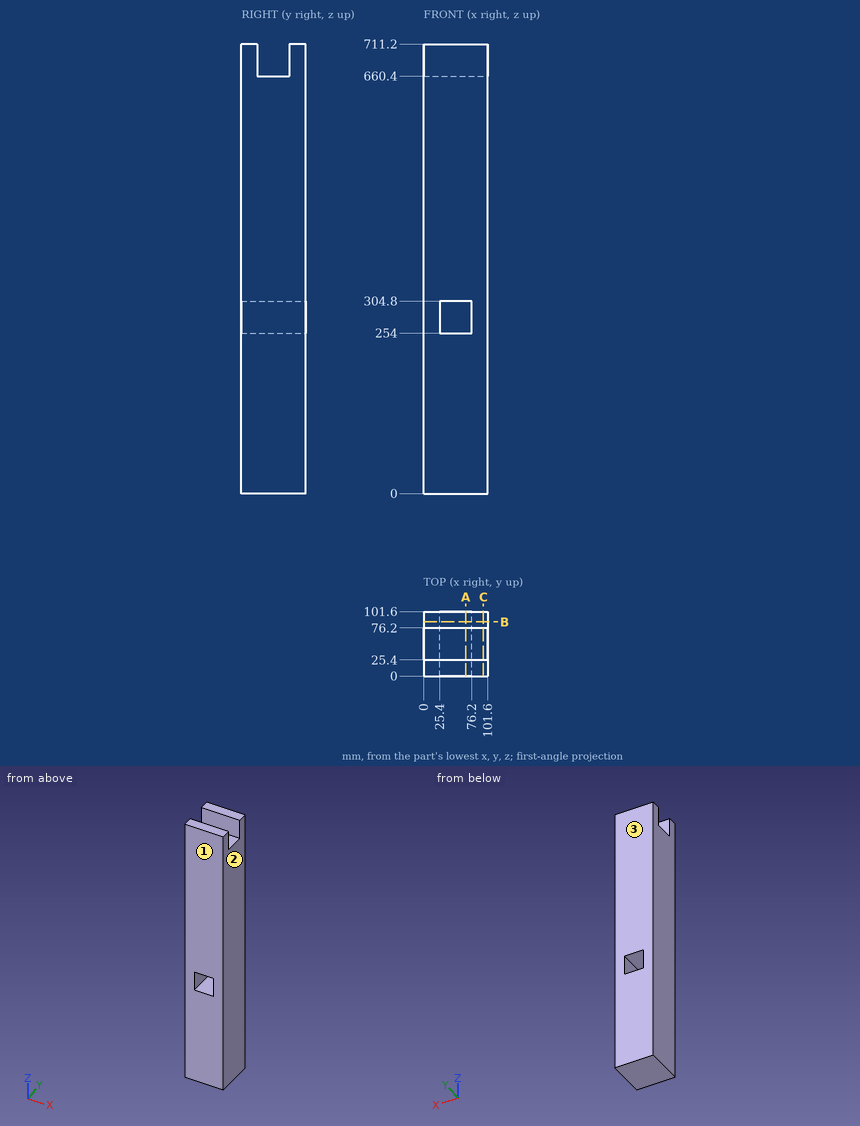
Part print with two shaded views. Sizes in mm from the minimum x, y, z corner. Round coordinates to 2 decimals unless told otherwise and drop trailing zeros. Loops run counter-clockwise (first coordinate to the right, second up) from the corner with the lowest first, then second, coordinate; pieces in that order, holes last. Notation, with made-up numbers: M 7.5,-4 L 27.5,-4 A12 cw 27.5,13 Z; hole C -30,15 d7. An arc over 180 degrees is marked long. Return JSON: item names as keys, results as strings. Group by question number.
(1) Saw through at B-B, the plane y = 85.5. List the corners of the cut face in (x, z), and give its area (3 significant figures).
(2) Mould opens along Y. For the marked faces 1, 2 and 3 say: +Y half, -Y half, draft (parallel to the pull), parting line (faces both ways), or undercut.
(3) Wall check: probe 1 along Z at (x, y) = (63, 79); probe 2 along Z at (x, y) = (55, 69); probe 3 along X at (y, z) = (58, 274). Give the ranges that are in metal, low to high. Write a range as [from, to].
(4) Saw through at A-A, the plane x = 67. List the corners of the cut face in (y, z).
(5) Drop a flat-ended pin along its axis: P1, Ø1.5, axis at x = 37.5, y = 40.5, coming from the +Z side. Give the stop position or say it passes through.
(6) Saw through at C-C, the plane x = 94.5. List the corners of the cut face in (y, z).
Answer list:
{
 "1": {"outline": "M 0,0 L 101.6,0 L 101.6,711.2 L 0,711.2 Z; hole M 25.4,254 L 76.2,254 L 76.2,304.8 L 25.4,304.8 Z", "area": "69,700 mm2"},
 "2": {"face 1": "-Y half", "face 2": "draft", "face 3": "+Y half"},
 "3": {"probe 1": "[0, 254], [304.8, 711.2]", "probe 2": "[0, 254], [304.8, 660.4]", "probe 3": "[0, 25.4], [76.2, 101.6]"},
 "4": {"outline": "M 0,0 L 101.6,0 L 101.6,254 L 0,254 Z; M 0,304.8 L 101.6,304.8 L 101.6,711.2 L 76.2,711.2 L 76.2,660.4 L 25.4,660.4 L 25.4,711.2 L 0,711.2 Z"},
 "5": {"P1": "z = 660.4"},
 "6": {"outline": "M 0,0 L 101.6,0 L 101.6,711.2 L 76.2,711.2 L 76.2,660.4 L 25.4,660.4 L 25.4,711.2 L 0,711.2 Z"}
}
